```python
from build123d import *

# Parameters (mm, degrees)
F0_R     = 2
F0_R_2   = 13.725453
F1_DEPTH = 7
F2_SIZE  = 2


with BuildPart() as f1:
    # F0 (on Top) → F1 (new body)
    with BuildSketch(Plane.XY):
        Polygon((5, 43.660253), (-5, 43.660253), (-7.886752, 43.660253), (-9.330152, 41.160211), (-14.330019, 32.500187), (-15.773503, 30), (-14.328388, 27.496988), (-9.330127, 18.839746), (-20.980762, -1.339746), (-30.980762, -1.339746), (-33.867513, -1.339746), (-35.310889, -3.839746), (-40.310889, -12.5), (-41.754264, -15), (-40.310888, -17.499999), (-35.310888, -26.160254), (-33.867512, -28.660255), (-30.980762, -28.660255), (-20.980762, -28.660255), (-18.094012, -28.660255), (-16.649425, -26.158157), (-11.650635, -17.5), (11.650635, -17.5), (16.650482, -26.159988), (18.094012, -28.660255), (20.980762, -28.660255), (30.980762, -28.660255), (33.867512, -28.660255), (35.310888, -26.160254), (40.309298, -17.502755), (41.754264, -15), (40.310625, -12.499543), (35.312513, -3.84256), (33.867513, -1.339746), (30.980762, -1.339746), (20.980762, -1.339746), (9.330127, 18.839746), (14.330123, 27.499994), (15.773503, 30), (14.329358, 32.501332), (9.330202, 41.160124), (7.886752, 43.660253), align=None)
        Polygon((-30.980762, -6.339746), (-20.980762, -6.339746), (-15.980762, -15), (-20.980762, -23.660254), (-30.980762, -23.660254), (-35.980762, -15), align=None, mode=Mode.SUBTRACT)
        with Locations((-11.607334, -13.425)):
            Circle(F0_R, mode=Mode.SUBTRACT)
        with Locations((-17.430058, -4.289746)):
            Circle(F0_R, mode=Mode.SUBTRACT)
        Circle(F0_R_2, mode=Mode.SUBTRACT)
        with Locations((12.430058, -12.95)):
            Circle(F0_R, mode=Mode.SUBTRACT)
        Polygon((20.980762, -23.660254), (15.980762, -15), (20.980762, -6.339746), (30.980762, -6.339746), (35.980762, -15), (30.980762, -23.660254), align=None, mode=Mode.SUBTRACT)
        with Locations((17.430058, -4.339746)):
            Circle(F0_R, mode=Mode.SUBTRACT)
        with Locations((-5, 17.239746)):
            Circle(F0_R, mode=Mode.SUBTRACT)
        Polygon((10, 30), (5, 21.339746), (-5, 21.339746), (-10, 30), (-5, 38.660254), (5, 38.660254), align=None, mode=Mode.SUBTRACT)
        with Locations((5, 17.239746)):
            Circle(F0_R, mode=Mode.SUBTRACT)
    extrude(amount=F1_DEPTH)

    # F2
    f2_edges = [f1.edges().sort_by_distance(p)[0] for p in [
        (-11.830127, 36.830127, 7),
        (0, 43.660253, 7),
        (-12.551815, 24.419873, 7),
        (11.830127, 36.830127, 7),
        (12.551815, 24.419873, 7),
        (15.155444, 8.75, 7),
        (27.424137, -1.339746, 7),
        (37.810888, -8.169873, 7),
        (37.810888, -21.830127, 7),
        (25.980762, -28.660255, 7),
        (14.872323, -23.080127, 7),
        (0, -17.5, 7),
        (-14.872323, -23.080127, 7),
        (-25.980762, -28.660255, 7),
        (-37.810888, -21.830127, 7),
        (-37.810888, -8.169873, 7),
        (-27.424137, -1.339746, 7),
        (-15.155444, 8.75, 7),
        (-27.424137, -1.339746, 0),
        (-37.810888, -8.169873, 0),
        (-37.810888, -21.830127, 0),
        (-25.980762, -28.660255, 0),
        (-14.872323, -23.080127, 0),
        (0, -17.5, 0),
        (14.872323, -23.080127, 0),
        (25.980762, -28.660255, 0),
        (37.810888, -21.830127, 0),
        (37.810888, -8.169873, 0),
        (27.424137, -1.339746, 0),
        (15.155444, 8.75, 0),
        (12.551815, 24.419873, 0),
        (11.830127, 36.830127, 0),
        (0, 43.660253, 0),
        (-11.830127, 36.830127, 0),
        (-12.551815, 24.419873, 0),
        (-15.155444, 8.75, 0),
    ]]
    chamfer(f2_edges, length=F2_SIZE)


solid = f1.part
```
Read the model definition and answer for the solid it produces. Units are mm, in the model's axes. A direction names the side the tool comes from. Round coordinates to 2 decimals unless told otherwise and drop trailing zeros. Write each loop counter-clockwise with the first axis right and the second up, starting at its lowest first coordinate (ties: lowest second). Pieces come first, ordered by that corner, then holes. Notation, with made-up numbers: (3, 41) - (11, 41) arc R33 cw to (11, 71) - close; hole circle Ø4 at (85, -20.5). An arc over 180 degrees is marked (long way). Use CSV: the item, a comma, the result in double quotes.
Q1. Find section D-D, the plane y = -20.5. Write down the section's boundary in (x, z), then the cut area to 3 significant figures.
Values:
outline,"(-38.58, 2) - (-36.27, 0) - (-32.81, 0) - (-32.81, 7) - (-36.27, 7) - (-38.58, 5) - close; (-19.16, 0) - (-15.69, 0) - (-13.38, 2) - (-13.38, 5) - (-15.69, 7) - (-19.16, 7) - close; (13.38, 2) - (15.69, 0) - (19.16, 0) - (19.16, 7) - (15.69, 7) - (13.38, 5) - close; (32.81, 0) - (36.27, 0) - (38.58, 2) - (38.58, 5) - (36.27, 7) - (32.81, 7) - close"
area,"143 mm²"
Q2. Find section C-C, the plane y = 24. Write down the section's boundary in (x, z).
Values:
outline,"(-12.31, 2) - (-10, 0) - (-6.54, 0) - (-6.54, 7) - (-10, 7) - (-12.31, 5) - close; (6.54, 0) - (10, 0) - (12.31, 2) - (12.31, 5) - (10, 7) - (6.54, 7) - close"
Q3. Find section B-B, the plane y = -10. Write down the section's boundary in (x, z), then the cut area to 3 significant figures.
Values:
outline,"(-38.87, 2) - (-36.56, 0) - (-33.09, 0) - (-33.09, 7) - (-36.56, 7) - (-38.87, 5) - close; (-18.87, 0) - (-9.4, 0) - (-9.4, 7) - (-18.87, 7) - close; (9.4, 0) - (18.87, 0) - (18.87, 7) - (9.4, 7) - close; (33.09, 0) - (36.56, 0) - (38.87, 2) - (38.87, 5) - (36.56, 7) - (33.09, 7) - close"
area,"204 mm²"
Q4. Determine the mould class of faces 1 (the flat face through (-26.75, -2.35, 0.99)), 2 (the flat face through (-0.2, -16.5, 6)), 3 (the flat face through (15.237, 8.609, 3.479)) for opening direction Y: +Y half, -Y half, draft (parallel to the pull), parting line (faces both ways), or undercut.
Values:
face 1,"+Y half"
face 2,"-Y half"
face 3,"undercut"
Q5. Each of these flat-tipped pins is pushed along its axis until it touches: pin 1 Ø6.5 at (x, y) = (17.43, -4.34) entering from +Z; pin 2 Ø2 at (x, z) = (28, 4.5) entering from +Y; pin 3 Ø2 at (x, y) = (-11.5, -4) entering from +Z; pin 4 Ø0.9 at (x, z) = (-3.5, 4) entering from -Y. Where does it stop, or does it pass through?
Values:
pin 1,"stops at z = 7"
pin 2,"stops at y = -1.34"
pin 3,"passes through"
pin 4,"stops at y = -17.5"
Q6. Straight lines are drawn through the part: line 1 along Y through (x, z) = (0, 4.25); line 2 along Y through (x, z) = (1, 6); line 3 along X through (y, z) = (16.5, 3). For each, find the intervals that lie inside material, in ascending order.
Values:
line 1,"y = -17.5 to -13.73, 13.73 to 21.34, 38.66 to 43.66"
line 2,"y = -16.5 to -13.69, 13.69 to 21.34, 38.66 to 42.66"
line 3,"x = -10.68 to -6.86, -3.14 to 3.14, 6.86 to 10.68"
Q7. A tool of negligible diameter and unlimited length cuts with its end or side. For faces 4 (the flat face through (-15.074, 8.891, 3.479)), 5 (the flat face through (-14.2, 8.4, 6)), 6 (the flat face through (-14.2, 8.4, 1)), 7 (the flat face through (7.535, 25.73, 3.451)), from which of +Z, -Z, +X, -X, +Y, -Y can it reach the whole face along a straight path? Write none if from no direction.
Values:
face 4,"+Z, -Z, -X"
face 5,"+Z, -X"
face 6,"-Z, -X"
face 7,"+Z, -Z"
Q8. Find section A-A, the plane x = -26.5. Write down the section's boundary in (y, z).
Values:
outline,"(-28.66, 2) - (-26.66, 0) - (-23.66, 0) - (-23.66, 7) - (-26.66, 7) - (-28.66, 5) - close; (-6.34, 0) - (-3.34, 0) - (-1.34, 2) - (-1.34, 5) - (-3.34, 7) - (-6.34, 7) - close"
